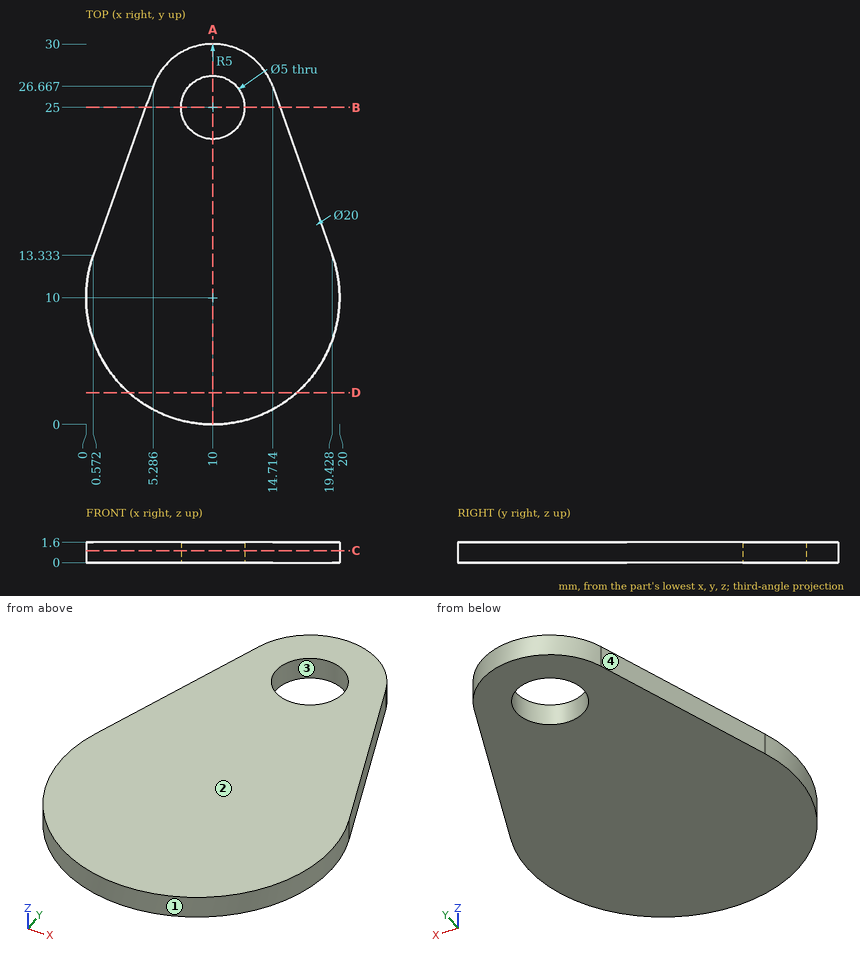
Design review of the part shown in the three views and the two pictorial views. Dimensions are in mm from the part's minimum x, y and z. Give positions to 0.01 mm unless a question says otherwise; leave off trailing zeros. Loops run counter-clockwise (first coordinate to the right, second up) from the corner with the lowest first, then second, coordinate; pieces in that order, holes last. Notation, with made-up numbers: (35, 70) - (54, 70) arc R21 cw to (54, 76) - close; hole circle Ø5 at (68.5, 65). An arc over 180 degrees is marked (long way). Write item = value, one per line.
1) Take a section at C-C on z = 0.95. State the section outline as (x, y) points.
Result sheet:
outline = (0.57, 13.33) arc R10 ccw (long way) to (19.43, 13.33) - (14.71, 26.67) arc R5 ccw to (5.29, 26.67) - close; hole circle Ø5 at (10, 25)
2) Draft analysis for pull direction X (two halves, no side actions). For the marked faces 1, 2, 3 and 4, state which applies: +X half, -X half, draft (parallel to the pull), parting line (faces both ways), or undercut.
Result sheet:
face_1 = parting line
face_2 = draft
face_3 = undercut
face_4 = -X half
3) To check wall thickness, follow line 1 (Y direction, x = 12, z = 0.6); line 2 (Y direction, x = 9, z = 0.15); line 3 (X direction, y = 25, z = 0.3). State the ranges of each line that lie inside material, in increasing order.
Result sheet:
line_1 = 0.2 to 23.5, 26.5 to 29.58
line_2 = 0.05 to 22.71, 27.29 to 29.9
line_3 = 4.7 to 7.5, 12.5 to 15.3
4) Take a section at B-B on y = 25. State the section outline as (x, z) points.
Result sheet:
outline = (4.7, 0) - (7.5, 0) - (7.5, 1.6) - (4.7, 1.6) - close; (12.5, 0) - (15.3, 0) - (15.3, 1.6) - (12.5, 1.6) - close
5) Take a section at D-D on y = 2.5. State the section outline as (x, z) points.
Result sheet:
outline = (3.39, 0) - (16.61, 0) - (16.61, 1.6) - (3.39, 1.6) - close
6) Clearance check with a flat-ended pin moving along its axis: pin 1 Ø3 at (x, y) = (10, 25) entering from +Z. State where the tip first meets the part, or that it passes through.
Result sheet:
pin_1 = through
7) Take a section at A-A on x = 10. State the section outline as (y, z) points.
Result sheet:
outline = (0, 0) - (22.5, 0) - (22.5, 1.6) - (0, 1.6) - close; (27.5, 0) - (30, 0) - (30, 1.6) - (27.5, 1.6) - close
